Can you work these out from the model? Positions are in its coordinate system, mm. Round coordinates to 2 decimals unless told otherwise and drop trailing zeros. Write each loop counter-clockwise with the first axis right and the second up, starting at its lowest first coordinate (ties: lowest second). Pieces come first, ordered by that corner, then holes. Notation, with made-up numbers: (-38, 57.5) -> (-12, 57.5) arc R17 ccw to (-12, 73.5) -> close; hole circle Ø9 at (9, 36). An arc over 180 degrees is marked (long way). Write item = value, one per line. Start each with the question number.
1) Imagine slicing it at A-A, the plane y = 277.5. Please give me the cut outline in (x, z).
2) I'm going to push a flat-ended pin straight in: pin 1 (4 mm diameter, centred on y = 158.75, z = 215.9, fed in from -X). Where does the tip first touch, or does it pass through?
3) If I drill on line 1 (Y direction, x = -325.5, z = 107.95) (3 decimals); line 2 (Y direction, x = -329, z = 323.85) (3 decimals); line 3 (Z direction, x = -329.5, y = 385.5), over which ranges is the centre line in solid material (lowest first)?
4) Imagine slicing it at B-B, the plane z = -245. Please give me the cut outline in (x, y), then the cut area to 3 significant figures.
5) Imagine slicing it at C-C, the plane x = -327. State how many separate pieces and enclosed holes the cut face has, then the cut area to 3 significant figures.
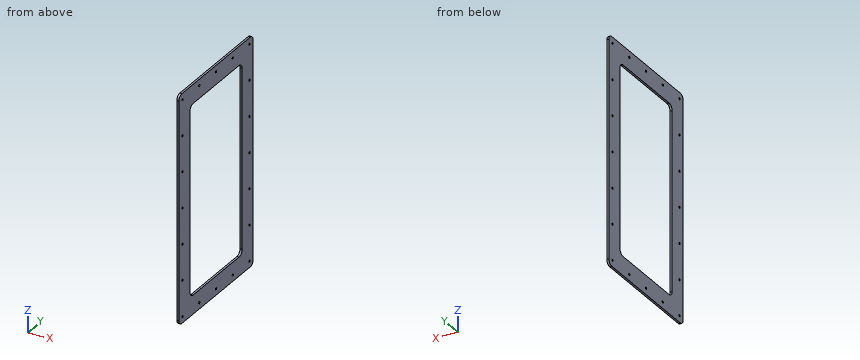
from build123d import *

# Parameters (mm, degrees)
BOSS_EXTRUDE1_START         = 12.7
SKETCH1_W                   = 685.8
SKETCH1_H                   = 381
SKETCH1_W_2                 = 571.5
SKETCH1_H_2                 = 266.7
BOSS_EXTRUDE1_DEPTH         = 6.35
F_1_4_0_25_DIAMETER_HOLE1_D = 6.35
LPATTERN2_COUNT             = 7
LPATTERN2_PITCH             = 107.95
LPATTERN2_COUNT_DIR2        = 5
LPATTERN2_PITCH_DIR2        = 85.725
FILLET1_R                   = 15.24


with BuildPart() as part:
    # Sketch1 → Boss-Extrude1 (new body)
    with BuildSketch(Plane.ZY.offset(311.15).offset(BOSS_EXTRUDE1_START)):
        with Locations((0, 330.2)):
            Rectangle(SKETCH1_W, SKETCH1_H)
        with Locations((0, 330.2)):
            Rectangle(SKETCH1_W_2, SKETCH1_H_2, mode=Mode.SUBTRACT)
    extrude(amount=BOSS_EXTRUDE1_DEPTH)

    # 1/4 (0.25) Diameter Hole1 (through all)
    with Locations(Plane.ZY.offset(330.2)):
        with Locations((-323.85, 158.75)):
            f_1_4_0_25_diameter_hole1 = Hole(F_1_4_0_25_DIAMETER_HOLE1_D / 2)

    # LPattern2: 1_4 _0.25_ Diameter Hole1 7 × 5, 15 skipped
    with Locations(*[(0, j * LPATTERN2_PITCH_DIR2, i * LPATTERN2_PITCH) for i in range(LPATTERN2_COUNT) for j in range(LPATTERN2_COUNT_DIR2) if (i, j) not in ((0, 0), (1, 1), (1, 2), (1, 3), (2, 1), (2, 2), (2, 3), (3, 1), (3, 2), (3, 3), (4, 1), (4, 2), (4, 3), (5, 1), (5, 2), (5, 3))]):
        add(f_1_4_0_25_diameter_hole1, mode=Mode.SUBTRACT)

    # Fillet1
    fillet1_edges = [part.edges().sort_by_distance(p)[0] for p in [
        (-327.025, 463.55, -285.75),
        (-327.025, 196.85, -285.75),
        (-327.025, 196.85, 285.75),
        (-327.025, 463.55, 285.75),
        (-327.025, 520.7, -342.9),
        (-327.025, 520.7, 342.9),
        (-327.025, 139.7, 342.9),
        (-327.025, 139.7, -342.9),
    ]]
    fillet(fillet1_edges, radius=FILLET1_R)


solid = part.part
Reported:
q1.outline = (-330.2, -342.9) -> (-323.85, -342.9) -> (-323.85, -285.75) -> (-330.2, -285.75) -> close; (-330.2, 285.75) -> (-323.85, 285.75) -> (-323.85, 342.9) -> (-330.2, 342.9) -> close
q2.pin_1 = through
q3.line_1 = 139.7 to 155.575, 161.925 to 196.85, 463.55 to 498.475, 504.825 to 520.7
q3.line_2 = 139.7 to 155.575, 161.925 to 241.3, 247.65 to 327.025, 333.375 to 412.75, 419.1 to 498.475, 504.825 to 520.7
q3.line_3 = -342.9 to -285.75, 285.75 to 342.9
q4.outline = (-330.2, 139.7) -> (-323.85, 139.7) -> (-323.85, 196.85) -> (-330.2, 196.85) -> close; (-330.2, 463.55) -> (-323.85, 463.55) -> (-323.85, 520.7) -> (-330.2, 520.7) -> close
q4.area = 726 mm²
q5.separate_pieces = 1
q5.enclosed_holes = 21
q5.area = 108,000 mm²
